For this review, take the finished solid that the model builds, in its own axes (mm). Face numbers are marked on the shaded views. A direction names the side the tool comes from. Round coordinates to 2 decimals unless told otherwise and drop trailing zeros. Write each loop counter-clockwise with the first axis right and the second up, starting at its lowest first coordinate (ties: lowest second). Pieces come first, ordered by that corner, then holes. Notation, with made-up numbers: (22, 1.25) -> (60, 1.25) arc R29 cw to (60, 38.25) -> close; hole circle Ø7 at (86, 61). An arc over 180 degrees is marked (long way). Write each question's results on one line, items separated by ' | '. Start each with the question number.
Item 1: Add section A-A (x = 0). State the section outline as (y, z) points, plus the area to 3 significant figures.
Item 2: Add section D-D (x = -26). State the section outline as (y, z) points, plus the area to 3 significant figures.
Item 3: Clearance check with flat-ended pins moving along their axes: pin 1 (12 mm diameter, centred on x = -43.5, z = 16, fed in from -Y); pin 2 (1.5 mm diameter, centred on x = 38, z = 8.5, fed in from +Y); pin 3 (5 mm diameter, centred on y = -34.5, z = 6, fed in from +X). State where each tip first meets the part, or that it passes through.
Item 4: The part is to be moulded in two halves that separate along X. For the marked faces 3, 4 and 5, say which applies: +X half, -X half, draft (parallel to the pull), parting line (faces both ways), or undercut.
Item 5: Tool access review of the marked faces 1 and 2: name each direction out of +Z, -Z, +X, -X, +Y, -Y from which nothing blocks a thin tool from reaching the whole face with its end or side.
Item 6: Add section B-B (z = 17.25). State the section outline as (x, y) points.
Item 7: To check wall thickness, follow line 1 along Y through (x, z) = (0, 20.75); line 2 along Y through (x, z) = (0, 12.5); line 3 along X through (y, z) = (31.5, 14.5). State the ranges of each line that lie inside material, in increasing order.
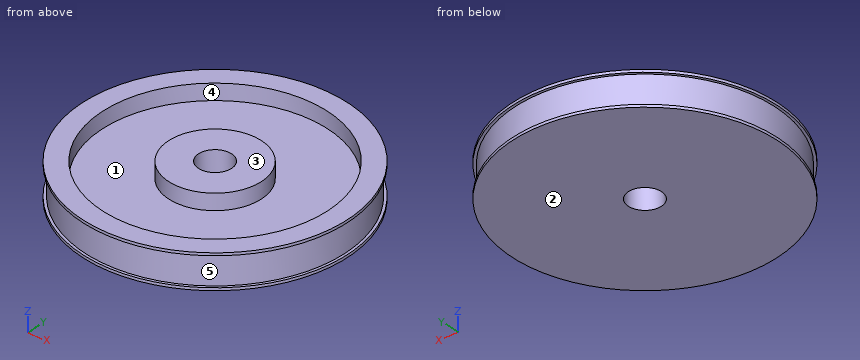
from build123d import *

# Parameters (mm, degrees)
SKETCH1_R           = 100
SKETCH1_R_2         = 12.5
BOSS_EXTRUDE1_DEPTH = 26
SKETCH3_OUTSIDE_W   = 258.808
SKETCH3_OUTSIDE_H   = 258.808
SKETCH3_OUTSIDE_R   = 98
CUT_EXTRUDE3_DEPTH  = 24
BOSS_EXTRUDE3_START = -2
SKETCH6_R           = 100
BOSS_EXTRUDE3_DEPTH = 2
SKETCH7_R           = 12.5
CUT_EXTRUDE6_DEPTH  = 144.791515744
SKETCH8_R           = 85
SKETCH8_R_2         = 35
CUT_EXTRUDE7_DEPTH  = 12


with BuildPart() as part:
    # Sketch1 → Boss-Extrude1 (new body)
    with BuildSketch(Plane.XY):
        with Locations(Location((0, 0, 0), (0, 0, 180))):
            Circle(SKETCH1_R)
        with Locations(Location((0, 0, 0), (0, 0, 180))):
            Circle(SKETCH1_R_2, mode=Mode.SUBTRACT)
    extrude(amount=BOSS_EXTRUDE1_DEPTH)

    # Sketch3 outside → Cut-Extrude3 (cut)
    with BuildSketch(Plane.XY.offset(26)):
        Rectangle(SKETCH3_OUTSIDE_W, SKETCH3_OUTSIDE_H)
        Circle(SKETCH3_OUTSIDE_R, mode=Mode.SUBTRACT)
    extrude(amount=-CUT_EXTRUDE3_DEPTH, mode=Mode.SUBTRACT)

    # Sketch6 → Boss-Extrude3 (add)
    with BuildSketch(Plane.XY.offset(26).offset(BOSS_EXTRUDE3_START)):
        with Locations(Location((0, 0, 0), (0, 0, 180))):
            Circle(SKETCH6_R)
    extrude(amount=BOSS_EXTRUDE3_DEPTH)

    # Sketch7 → Cut-Extrude6 (cut, through all)
    with BuildSketch(Plane(origin=(0, 0, 0), x_dir=(-1, 0, 0), z_dir=(0, 0, -1))):
        Circle(SKETCH7_R)
    extrude(amount=-CUT_EXTRUDE6_DEPTH, mode=Mode.SUBTRACT)

    # Sketch8 → Cut-Extrude7 (cut)
    with BuildSketch(Plane.XY.offset(26)):
        Circle(SKETCH8_R)
        Circle(SKETCH8_R_2, mode=Mode.SUBTRACT)
    extrude(amount=-CUT_EXTRUDE7_DEPTH, mode=Mode.SUBTRACT)


solid = part.part
Responses:
1) outline: (-100, 0) -> (-12.5, 0) -> (-12.5, 26) -> (-35, 26) -> (-35, 14) -> (-85, 14) -> (-85, 26) -> (-100, 26) -> (-100, 24) -> (-98, 24) -> (-98, 2) -> (-100, 2) -> close; (12.5, 0) -> (100, 0) -> (100, 2) -> (98, 2) -> (98, 24) -> (100, 24) -> (100, 26) -> (85, 26) -> (85, 14) -> (35, 14) -> (35, 26) -> (12.5, 26) -> close | area: 3,260 mm^2
2) outline: (-96.56, 0) -> (96.56, 0) -> (96.56, 2) -> (94.49, 2) -> (94.49, 24) -> (96.56, 24) -> (96.56, 26) -> (80.93, 26) -> (80.93, 14) -> (23.43, 14) -> (23.43, 26) -> (-23.43, 26) -> (-23.43, 14) -> (-80.93, 14) -> (-80.93, 26) -> (-96.56, 26) -> (-96.56, 24) -> (-94.49, 24) -> (-94.49, 2) -> (-96.56, 2) -> close | area: 3,550 mm^2
3) pin 1: stops at y = -90.54 | pin 2: stops at y = 90.64 | pin 3: stops at x = 92.63
4) face 3: draft | face 4: undercut | face 5: parting line
5) face 1: +Z | face 2: -Z, +X, -X, +Y, -Y
6) outline: circle Ø196 at (0, 0); circle Ø70 at (0, 0); hole circle Ø170 at (0, 0); hole circle Ø25 at (0, 0)
7) line 1: y = -98 to -85, -35 to -12.5, 12.5 to 35, 85 to 98 | line 2: y = -98 to -12.5, 12.5 to 98 | line 3: x = -92.8 to -78.95, -15.26 to 15.26, 78.95 to 92.8
